CAD build for the part. Positions are in the model's coordinates, mm. Face numbers are marked on the shaded views. A direction names the side the tool comes from. Coordinates: 2 decimals unless noted, no trailing zeros. Order: outer loops, then holes, each group sorted by start corner. A loop starts at its lowest first (then second) coordinate and runs counter-clockwise, first axis right, second up. Notation, with made-up numbers: (71.25, 58) - (101.25, 58) arc R17 ccw to (101.25, 74) - close; hole circle Ø1 at (5, 4.5). An arc over 180 degrees is marked (long way). Return JSON: item names as keys, results as strings.
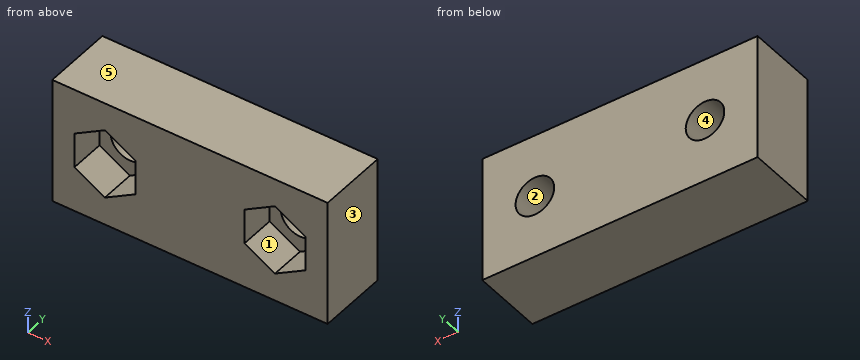
Solid Edge part; units mm, degrees
sketch "Sketch1" plane through (0, 0, 0) normal (0, -1, 0) x (1, 0, 0)
  circle A0 centre (-6.3238, 0) radius 2.2
  line L0 (-31.7238, 7.2) -> (-0.3238, 7.2)
  line L1 (-0.3238, 7.2) -> (-0.3238, -7.2)
  line L2 (-0.3238, -7.2) -> (-31.7238, -7.2)
  line L3 (-31.7238, -7.2) -> (-31.7238, 7.2)
  circle A1 centre (-25.7238, 0) radius 2.2
  dimension "D1" = 25.7238
  dimension "D2" = 25.7238
  dimension "D3" = 6.3238
extrude "Protrusion1" add sketch "Sketch1" along normal blind 8
sketch "Sketch2" plane through (-14.9238, -8, 0) normal (0, -1, 0) x (1, 0, 0)
  line L0 (-14.2641, -2) -> (-14.2641, 2)
  line L1 (-14.2641, 2) -> (-10.8, 4)
  line L2 (-10.8, 4) -> (-7.3359, 2)
  line L3 (-7.3359, 2) -> (-7.3359, -2)
  line L4 (-7.3359, -2) -> (-10.8, -4)
  line L5 (-10.8, -4) -> (-14.2641, -2)
extrude "ExtrudedCutout_1" cut sketch "Sketch2" against normal blind 4
mirror "Mirror1" about plane through (-16.0238, -4, 0) normal (-1, 0, 0) of "ExtrudedCutout_1"
Item 1: Which spindle directions (+Z, -Z, +X, -X, +Y, -Y) get a long thin tool onto all of the face, cutting with end or side? Do the marked faces 1 and 2. Say none if no direction does.
Findings below:
{"face 1": "-Y", "face 2": "+Y, -Y"}
Item 2: Band-saw the part on A-A, the plane z = 0. List the corners of the cut face in (x, y), then the cut area to 3 significant figures.
Findings below:
{"outline": "(-31.72, -8) - (-29.19, -8) - (-29.19, -4) - (-27.92, -4) - (-27.92, 0) - (-31.72, 0) - close; (-23.52, -4) - (-22.26, -4) - (-22.26, -8) - (-9.79, -8) - (-9.79, -4) - (-8.52, -4) - (-8.52, 0) - (-23.52, 0) - close; (-4.12, -4) - (-2.86, -4) - (-2.86, -8) - (-0.32, -8) - (-0.32, 0) - (-4.12, 0) - close", "area": "161 mm²"}
Item 3: Wall check: L1, parallel to X at y = -1.85, z = 0; L2, parallel to X at y = -6.5, z = -0.75; L3, parallel to Y at x = -25, z = -2.75. Give the ranges that are in metal, low to high. Write a range as [from, to].
Findings below:
{"L1": "x = [-31.72, -27.92], [-23.52, -8.52], [-4.12, -0.32]", "L2": "x = [-31.72, -29.19], [-22.26, -9.79], [-2.86, -0.32]", "L3": "y = [-4, 0]"}
Item 4: Band-saw the part on D-D, the plane y = -3. List the corners of the cut face in (x, z).
Findings below:
{"outline": "(-31.72, -7.2) - (-0.32, -7.2) - (-0.32, 7.2) - (-31.72, 7.2) - close; hole circle Ø4.4 at (-25.72, 0); hole circle Ø4.4 at (-6.32, 0)"}
Item 5: Mould opens along X. For the marked faces 3, 4 and 5 say: released by +X, released by -X, zero draft, split by the parting line, or undercut.
Findings below:
{"face 3": "released by +X", "face 4": "undercut", "face 5": "zero draft"}
Item 6: Band-saw the part on C-C, the plane x = -4.5. List the corners of the cut face in (y, z), then the cut area to 3 significant figures.
Findings below:
{"outline": "(-8, -7.2) - (0, -7.2) - (0, -1.23) - (-4, -1.23) - (-4, -2.95) - (-8, -2.95) - close; (-8, 2.95) - (-4, 2.95) - (-4, 1.23) - (0, 1.23) - (0, 7.2) - (-8, 7.2) - close", "area": "81.8 mm²"}
Item 7: Band-saw the part on B-B, the plane y = -4.75. List the corners of the cut face in (x, z), then the cut area to 3 significant figures.
Findings below:
{"outline": "(-31.72, -7.2) - (-0.32, -7.2) - (-0.32, 7.2) - (-31.72, 7.2) - close; hole (-29.19, -2) - (-25.72, -4) - (-22.26, -2) - (-22.26, 2) - (-25.72, 4) - (-29.19, 2) - close; hole (-9.79, -2) - (-6.32, -4) - (-2.86, -2) - (-2.86, 2) - (-6.32, 4) - (-9.79, 2) - close", "area": "369 mm²"}
